Here's how the part is built. I have some questions about the finished solid (model axes, mm). A direction names the side the tool comes from. Round coordinates to 2 decimals unless told otherwise and drop trailing zeros. Order: outer loops, then holes, each group sorted by start corner. A loop starts at its lowest first (then second) coordinate and runs counter-clockwise, first axis right, second up. Notation, with made-up numbers: M -13,-10.75 L 3,-10.75 A7 cw 3,1.25 Z; hole C -16.75,38 d2. An arc over 180 degrees is marked long. Write item = value, one per line. Start each with the question number.
Item 1: I want a section at C-C, the plane x = 30.5. List the corners of the cut face in (y, z) for me.
Item 2: Please list where these lines run through material, in increasing order: L1, parallel to Z at x = 48.5, y = 0; L2, parallel to X at y = -36, z = 2; L3, parallel to Y at x = 23, z = 21.5.
Item 3: For faces 3 (the face through (47, 13, 22)), 4 (the face through (40, 0, 8.5)), 5 (the face through (43, 0, 6)), which set-ups out of +Z, -Z, +X, -X, +Y, -Y let a thin tool reach every point of the face, with its end or its side?
Item 4: We'd pull the mould along Y, two halves only. Please class faces 1 (the face through (45.986, -8.554, 24.817)), 2 (the face through (27.115, 20.765, 39.923)): pulls with the +Y half, pulls with the -Y half, needs draft (parallel to the pull), parting line crosses it, or undercut.
Item 5: I'm going to push flat-ended pins straight in: P1, Ø2, axis at x = 46.5, y = -22, coming from the -Z side; P2, Ø3, axis at y = -31.5, z = 3, coming from the +X side; P3, Ø5.5, axis at y = -10.5, z = -22.5, coming from the -X side; P4, Ø14.5, axis at y = -32.5, z = -14, coming from the +X side. Where does each tip first touch, or does it pass through?
Item 6: I want a section at B-B, the plane y = 0. List the corners of the cut face in (x, z) for me.
Item 7: I want a section at A-A, the plane z = -22.5. List the corners of the cut face in (x, y) for me, plus the area to 3 significant figures.
Autodesk Inventor part; units mm, degrees
ref_plane "РабПлоскость1" through (45, 0, 0) normal (1, 0, 0) x (0, 0, -1)
ref_plane "YZ Plane" through (0, 0, 0) normal (1, 0, 0) x (0, 1, 0)
ref_plane "XZ Plane" through (0, 0, 0) normal (0, 1, 0) x (-1, 0, 0)
sketch "Эскиз1" plane through (0, 0, 0) normal (1, 0, 0) x (0, 1, 0)
  circle A0 centre (0, 0) radius 45
  circle A1 centre (0, 0) radius 40
  dimension "d0" = 90
  dimension "d1" = 5
extrude "Выдавливание1" add sketch "Эскиз1" along normal blind 55
ref_plane "РабПлоскость1" through (45, 0, 0) normal (1, 0, 0) x (0, 0, -1)
sketch "Эскиз2" plane through (45, 0, 0) normal (1, 0, 0) x (0, 0, -1)
  circle A0 centre (0, 0) radius 40
  circle A1 centre (0, 0) radius 35
  dimension "d5" = 5
extrude "Выдавливание2" add sketch "Эскиз2" against normal blind 2
sketch "Эскиз3" plane through (45, 0, 0) normal (1, 0, 0) x (0, 0, -1)
  circle A0 centre (0, 0) radius 6
  circle A1 centre (0, 0) radius 16
  circle A2 centre (0, 0) radius 35
  dimension "d19" = 12
  dimension "d20" = 32
extrude "Выдавливание3" add sketch "Эскиз3" against normal blind 4 contours A1
sketch "Эскиз4" plane through (45, 0, 0) normal (1, 0, 0) x (0, 0, -1)
  line L0 (-5, 42) -> (5, 42)
  line L1 (5, 42) -> (5, 11.4564)
  line L2 (-5, 11.4564) -> (-5, 42)
  line L3 (0, 0) -> (0, 36.2372) construction
  arc A0 (5, 11.4564) -> (-5, 11.4564) centre (0, 0) ccw
  dimension "d32" = 10
  dimension "d33" = 25
  dimension "d34" = 42
extrude "Выдавливание4" add sketch "Эскиз4" along normal blind 2
fillet "Сопряжение1" radius 1 5 edges at (46, 11.4564, -5) (46, 11.4564, 5) (47, 25.5714, 5) (47, 12.5, 0) (47, 25.5714, -5)
pattern_circular "Круговой массив1" count 6 over 360 about axis through (45, 0, 0) along (-1, 0, 0) of "Выдавливание4"
sketch "Эскиз5" plane through (41, 0, 0) normal (-1, 0, 0) x (0, 0, 1)
  line L0 (0, 9.815) -> (8.5, 4.9075)
  line L1 (8.5, 4.9075) -> (8.5, -4.9075)
  line L2 (8.5, -4.9075) -> (0, -9.815)
  line L3 (0, -9.815) -> (-8.5, -4.9075)
  line L4 (-8.5, -4.9075) -> (-8.5, 4.9075)
  line L5 (-8.5, 4.9075) -> (0, 9.815)
  circle A0 centre (0, 0) radius 16
  circle A1 centre (0, 0) radius 16
  dimension "d41" = 17
extrude "Выдавливание5" add sketch "Эскиз5" along normal blind 3
properties part number "КВ33-AN1-01-02-Диск"
Filled in:
q1.outline = C 0,0 d90; hole C 0,0 d80
q2.L1 = -45 to -40, 40 to 45
q2.L2 = 43 to 47
q2.L3 = -39.53 to -33.73, 33.73 to 39.53
q3.face_3 = +X
q3.face_4 = -X
q3.face_5 = +X, -X
q4.face_1 = undercut
q4.face_2 = parting line crosses it
q5.P1 = -39.8
q5.P2 = 47
q5.P3 = 45
q5.P4 = 55
q6.outline = M 0,-45 L 55,-45 L 55,-40 L 45,-40 L 45,-35 L 43,-35 L 43,-40 L 0,-40 Z; M 0,40 L 43,40 L 43,35 L 45,35 L 45,40 L 55,40 L 55,45 L 0,45 Z; M 38,-16 L 45,-16 L 45,-6 L 41,-6 L 41,-8.5 L 38,-8.5 Z; M 38,8.5 L 41,8.5 L 41,6 L 45,6 L 45,16 L 38,16 Z
q7.outline = M 0,-38.97 L 55,-38.97 L 55,-33.07 L 45,-33.07 L 45,-26.81 L 43,-26.81 L 43,-33.07 L 0,-33.07 Z; M 0,33.07 L 43,33.07 L 43,26.81 L 45,26.81 L 45,33.07 L 55,33.07 L 55,38.97 L 0,38.97 Z; M 45,-18.76 L 47,-18.76 L 47,-7.22 L 45,-7.22 Z; M 45,7.22 L 47,7.22 L 47,18.76 L 45,18.76 Z
q7.area = 720 mm^2
